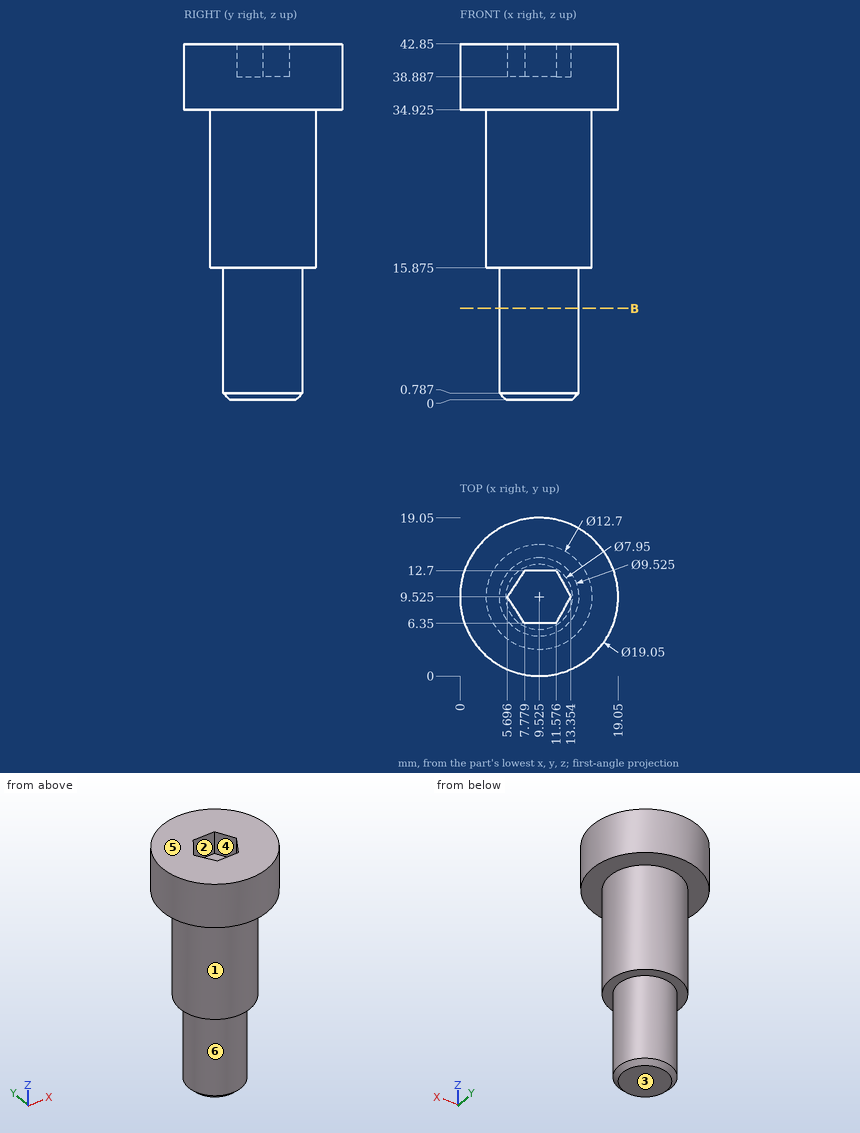
Print and shaded views of the part. All mm, measured from the part's lowest x, y and z. A direction names the side the tool comes from. Round coordinates to 2 decimals unless told otherwise and drop trailing zeros. Write each loop counter-clockwise with the first axis right and the second up, starting at its lowest first coordinate (ties: lowest second). Pieces come first, ordered by that corner, then holes. Notation, with made-up numbers: (-23.5, -40) - (15.5, -40) arc R27 ccw to (15.5, -3) - close; hole circle Ø1 at (-8, 37). An arc over 180 degrees is marked (long way). One line per item, written item: value.
(1) Cut at B-B, the plane z = 11. Give the cut face in (x, y) (1 decimal).
Values follow:
outline: circle Ø9.5 at (9.5, 9.5)
(2) Two-plate mould, pull along Y, no slides. Class the marked faces 1, 2 and 3: pulls with the +Y half, pulls with the -Y half, needs draft (parallel to the pull), parting line crosses it, or undercut.
Values follow:
face 1: parting line crosses it
face 2: undercut
face 3: needs draft
(3) Wall check: probe 1 along Y at (x, z) = (9.5, 30.5) (1 decimal); probe 2 along X at (y, z) = (8.5, 40.5) (1 decimal). Give the ranges that are in metal, low to high.
Values follow:
probe 1: y = 3.2 to 15.9
probe 2: x = 0.1 to 6.4, 12.8 to 19
(4) 3-axis set-ups, long thin cutter, end or side, ignore diameter. For the marked faces 4, 5 and 6: which of +Z, -Z, +X, -X, +Y, -Y reach the whole face in a straight line?
Values follow:
face 4: +Z
face 5: +Z, +X, -X, +Y, -Y
face 6: -Z
(5) Drop flat-ended pins along their axis: P1, Ø1, axis at x = 8, z = 15.5, coming from the +Y side; P2, Ø6, axis at x = 13, z = 28, coming from the +Y side; P3, Ø8, axis at y = 16.5, z = 10, coming from the -X side (1 decimal). Give the stop position or say it passes through.
Values follow:
P1: stops at y = 15.76
P2: stops at y = 15.86
P3: stops at x = 5.8
